Check sheet for the modelled part. Datum: model origin and axes. Units: mm. Round coordinates to 2 decimals unless told otherwise and drop trailing zeros. Order: outer loops, then holes, each group sorted by start corner. A loop starts at its lowest first (then second) coordinate and runs counter-clockwise, first axis right, second up.
```python
from build123d import *

# Parameters (mm, degrees)
F0_W     = 600
F0_H     = 350
F1_DEPTH = 1
F2_W     = 1
F2_H     = 350
F3_DEPTH = 30
F4_R     = 2.888971
F5_DEPTH = 735
F6_W     = 500
F6_H     = 1
F7_DEPTH = 10


with BuildPart() as f1:
    # F0 (on Top) → F1 (new body)
    with BuildSketch(Plane.XY):
        with Locations((3.478525, 2.822831)):
            Rectangle(F0_W, F0_H)
    extrude(amount=F1_DEPTH)

    # F2 (on face) → F3 (join)
    with BuildSketch(Plane.XY.offset(1)):
        with Locations((-296.021475, 2.822831)):
            Rectangle(F2_W, F2_H)
        with Locations((302.978525, 2.822831)):
            Rectangle(F2_W, F2_H)
    extrude(amount=F3_DEPTH)

    # F4 (on face) → F5 (cut)
    with BuildSketch(Plane(origin=(-296.521475, 0, 0), x_dir=(0, -1, 0), z_dir=(-1, 0, 0))):
        with Locations((-162.822831, 15)):
            Circle(F4_R)
    extrude(amount=-F5_DEPTH, mode=Mode.SUBTRACT)

    # F6 (on face) → F7 (join)
    with BuildSketch(Plane.XY.offset(1)):
        with Locations((3.478525, 77.322831)):
            Rectangle(F6_W, F6_H)
        with Locations((3.478525, -71.677169)):
            Rectangle(F6_W, F6_H)
    extrude(amount=F7_DEPTH)


solid = f1.part
```
Item 1: Release check for a two-part mould opening along X. For faces 1 (the flat face through (303.479, 0, 15)), 2 (the flat face through (302.479, 0, 16)), 3 (the flat face through (-1, 5, 0)), 4 (the flat face through (-295.521, 0, 16)) record: released by +X, released by -X, zero draft, split by the parting line, or undercut.
Answer:
face 1: released by +X
face 2: undercut
face 3: zero draft
face 4: undercut
Item 2: Scan lines: line 1 along X through (y, z) = (50, 29.5); line 2 along Y through (x, z) = (67, 5); line 3 along X through (y, z) = (77.5, 6.5). Record each from-to range of solid material in increasing order.
Answer:
line 1: x = -296.52 to -295.52, 302.48 to 303.48
line 2: y = -72.18 to -71.18, 76.82 to 77.82
line 3: x = -296.52 to -295.52, -246.52 to 253.48, 302.48 to 303.48
Item 3: Sectioned sample at A-A (x = 19). Record the cut outline in (y, z).
Answer:
outline: (-172.18, 0) - (177.82, 0) - (177.82, 1) - (77.82, 1) - (77.82, 11) - (76.82, 11) - (76.82, 1) - (-71.18, 1) - (-71.18, 11) - (-72.18, 11) - (-72.18, 1) - (-172.18, 1) - close
Item 4: Sectioned sample at B-B (y = 104.5). Record the cut outline in (x, z).
Answer:
outline: (-296.52, 0) - (303.48, 0) - (303.48, 31) - (302.48, 31) - (302.48, 1) - (-295.52, 1) - (-295.52, 31) - (-296.52, 31) - close
Item 5: Go/stop test with flat-tipped pins: P1, Ø0.8, axis at x = 7.5, y = -71.5, coming from the +Z side; P2, Ø3, axis at x = -80.5, z = 8, coming from the -Y side; P3, Ø1, axis at x = 90, y = -84.5, coming from the +Z side; P4, Ø12, axis at x = -124, z = 19, coming from the -Y side. Record where each tip stops, or that it passes through.
Answer:
P1: stops at z = 11
P2: stops at y = -72.18
P3: stops at z = 1
P4: passes through
